```python
from build123d import *

# Parameters (mm, degrees)
SKETCH4_R          = 25.4
CUT_EXTRUDE1_DEPTH = 2.54


with BuildPart() as part:
    # Sketch3 → Revolve1 (revolve)
    with BuildSketch(Plane(origin=(0, 0, 0), x_dir=(0, 0, -1), z_dir=(1, 0, 0)), mode=Mode.PRIVATE) as revolve1_sk:
        with BuildLine():
            Line((0.49609375, 36.5125), (-0.49609375, 36.5125))
            Line((-0.49609375, 36.5125), (-0.49609375, 35.2980625))
            ThreePointArc((-0.49609375, 35.2980625), (-0.53338976, 34.535400038), (-0.644921875, 33.780015625))
            ThreePointArc((-0.644921875, 33.780015625), (-0.75645399, 33.024631212), (-0.79375, 32.26196875))
            Line((-0.79375, 32.26196875), (-0.79375, 18.70075))
            ThreePointArc((-0.79375, 18.70075), (-0.756233853, 18.289154795), (-0.644921875, 17.891125))
            ThreePointArc((-0.644921875, 17.891125), (-0.533609897, 17.493095205), (-0.49609375, 17.0815))
            Line((-0.49609375, 17.0815), (-0.49609375, 16.271875))
            Line((-0.49609375, 16.271875), (0.49609375, 16.271875))
            Line((0.49609375, 16.271875), (0.49609375, 17.0815))
            ThreePointArc((0.49609375, 17.0815), (0.533609897, 17.493095205), (0.644921875, 17.891125))
            ThreePointArc((0.644921875, 17.891125), (0.756233853, 18.289154795), (0.79375, 18.70075))
            Line((0.79375, 18.70075), (0.79375, 32.26196875))
            ThreePointArc((0.79375, 32.26196875), (0.75645399, 33.024631212), (0.644921875, 33.780015625))
            ThreePointArc((0.644921875, 33.780015625), (0.53338976, 34.535400038), (0.49609375, 35.2980625))
            Line((0.49609375, 35.2980625), (0.49609375, 36.5125))
        make_face()
    revolve(revolve1_sk.sketch.rotate(Axis((0, 0, -0.79375), (0, 0, 1)), 90), axis=Axis((0, 0, -0.79375), (0, 0, 1)))

    # Sketch4 → Cut-Extrude1 (cut)
    with BuildSketch(Plane.XY.offset(0.79375)):
        Circle(SKETCH4_R)
    extrude(amount=-CUT_EXTRUDE1_DEPTH, mode=Mode.SUBTRACT)


solid = part.part
```
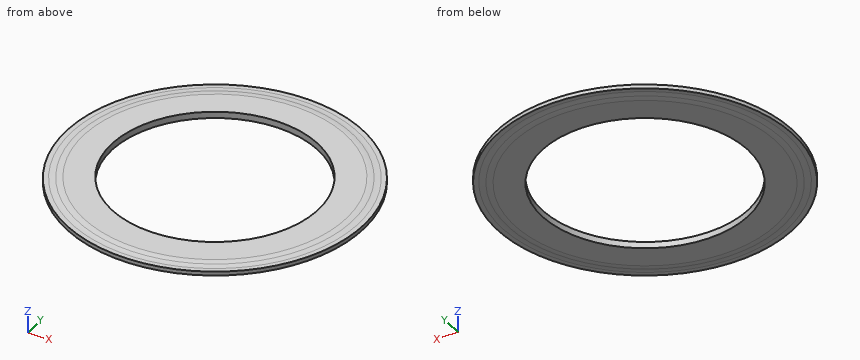
The model under review builds one solid part; all positions refer to its coordinate system, in mm. Give positions to 0.01 mm unless a question says otherwise; leave off trailing zeros. Write each loop counter-clockwise with the first axis right and the second up, starting at its lowest first coordinate (ties: lowest second). Pieces come first, ordered by that corner, then holes. Notation, with made-up numbers: (-14.5, 27) -> (28.5, 27) arc R18 cw to (28.5, 42) -> close; hole circle Ø8 at (-18.75, 60.5). An arc over 180 degrees is marked (long way). Put each result on its own line as item: value.
(1) To check wall thickness, follow probe 1 along Y at (x, z) = (0, -0.45); probe 2 along Z at (x, y) = (30.5, -11.5). State the ranges of each line that lie inside material, in increasing order. Write a range as from..to.
Results are:
probe 1: -36.51..-25.4, 25.4..36.51
probe 2: -0.79..0.79
(2) For pin 1 Ø22 at (x, y) = (0, 3.5) entering from +Z, flat-tipped, find the tip position at first contact; note if it passes through.
Results are:
pin 1: through
(3) We need section A-A, the plane z = 0.1. Give the boundary of the cut face in (x, y) (1 decimal), and give its area (3 significant figures).
Results are:
outline: circle Ø73 at (0, 0); hole circle Ø50.8 at (0, 0)
area: 2,160 mm²
